Check sheet for the modelled part. Datum: model origin and axes. Units: mm. A direction names the side the tool comes from. Coordinates: 2 decimals unless noted, no trailing zeros. Write each loop counter-clockwise with the first axis right and the second up, starting at its lowest first coordinate (ties: lowest second). Pieces come first, ordered by that corner, then holes. Notation, with made-up numbers: (13.5, 18) - (61.5, 18) arc R14 ccw to (61.5, 41) - close; hole circle Ø7 at (20.5, 50.5). An arc over 180 degrees is marked (long way). Use one line per item in the form item = value. Start each with the question number.
1. Cross-section at A-A on y = 1.75. Give the number of separate pieces and of enclosed holes in the cut face, then the cut area to 3 significant figures.
2. Cross-section at B-B on y = 5.5. Record the boundary of the cut face in (x, z).
3. Scan lines: line 1 along Z through (x, y) = (-6, 1.5); line 2 along Z through (x, y) = (0, -0.6); line 3 along Y through (x, z) = (5.75, -6.5). Record each from-to range of solid material in increasing order.
4. Tool access check on faces 4 (the face through (1, 6, -13)), 5 (the face through (-0.434, -0.493, -11.348)), 6 (the face through (8.225, 1.479, -12.585)). Record the directions out of +Z, -Z, +X, -X, +Y, -Y that give a thin tool (end or side, any length) a straight path to the whole face; none if there is none.
5. Draft check along Z on faces 1 (the face through (5, 0, -11)), 2 (the face through (5.624, 1.479, -19.706)), 3 (the face through (-9.126, 1.232, -6.302)). Enter one of: +Z half, -Z half, draft (parallel to the pull), parting line (faces both ways), or undercut.
6. Go/stop test with flat-tipped pins: pin 1 Ø1.7 at (x, z) = (5.66, -18.96) entering from +Y; pin 2 Ø2 at (x, y) = (-3.5, 5) entering from +Z; pin 3 Ø0.6 at (y, z) = (6, -13.5) entering from +X. Record where each tip stops, or that it passes through.
```python
from build123d import *

# Parameters (mm, degrees)
CROQUIS1_R              = 11.5
SALIENTE_EXTRUIR1_DEPTH = 3
CROQUIS1_9_R            = 0.75
CORTAR_EXTRUIR2_DEPTH   = 3
MATRIZC2_COUNT          = 8
SALIENTE_EXTRUIR2_START = 3
CROQUIS1_11_R           = 5
SALIENTE_EXTRUIR2_DEPTH = 1.5
SALIENTE_EXTRUIR3_START = 4.5
CROQUIS1_12_R           = 2
SALIENTE_EXTRUIR3_DEPTH = 3
REDONDEO1_R             = 0.5
CROQUIS1_13_R           = 5
CROQUIS1_13_R_2         = 2
SALIENTE_EXTRUIR4_DEPTH = 1


with BuildPart() as part:
    # Croquis1 → Saliente-Extruir1 (new body)
    with BuildSketch(Plane(origin=(0, 0, 0), x_dir=(1, 0, 0), z_dir=(0, 1, 0))):
        with Locations((0, 13.3)):
            Circle(CROQUIS1_R)
    extrude(amount=SALIENTE_EXTRUIR1_DEPTH)

    # Croquis1<9> → Cortar-Extruir2 (cut)
    with BuildSketch(Plane(origin=(0, 0, 0), x_dir=(1, 0, 0), z_dir=(0, 1, 0))):
        with Locations((0, 21.3)):
            Circle(CROQUIS1_9_R)
    cortar_extruir2 = extrude(amount=CORTAR_EXTRUIR2_DEPTH, mode=Mode.SUBTRACT)

    # MatrizC2: Cortar-Extruir2 ×8 about axis
    matrizc2_axis = Axis((0, 0, -13.3), (0, 1, 0))
    for i in range(1, MATRIZC2_COUNT):
        add(cortar_extruir2.rotate(matrizc2_axis, i * 360 / MATRIZC2_COUNT), mode=Mode.SUBTRACT)

    # Croquis1<11> → Saliente-Extruir2 (add)
    with BuildSketch(Plane(origin=(0, 0, 0), x_dir=(1, 0, 0), z_dir=(0, 1, 0)).offset(SALIENTE_EXTRUIR2_START)):
        with Locations((0, 13.3)):
            Circle(CROQUIS1_11_R)
    extrude(amount=SALIENTE_EXTRUIR2_DEPTH)

    # Croquis1<12> → Saliente-Extruir3 (add)
    with BuildSketch(Plane(origin=(0, 0, 0), x_dir=(1, 0, 0), z_dir=(0, 1, 0)).offset(SALIENTE_EXTRUIR3_START)):
        with Locations((0, 13.3)):
            Circle(CROQUIS1_12_R)
        Polygon((1, 12.722649731), (1, 13.877350269), (0, 14.454700538), (-1, 13.877350269), (-1, 12.722649731), (0, 12.145299462), align=None, mode=Mode.SUBTRACT)
    extrude(amount=SALIENTE_EXTRUIR3_DEPTH)

    # Redondeo1
    redondeo1_edges = [part.edges().sort_by_distance(p)[0] for p in [
        (-11.5, 3, -13.3),
        (-5, 4.5, -13.3),
        (-2, 7.5, -13.3),
    ]]
    fillet(redondeo1_edges, radius=REDONDEO1_R)

    # Croquis1<13> → Saliente-Extruir4 (add)
    with BuildSketch(Plane(origin=(0, 0, 0), x_dir=(1, 0, 0), z_dir=(0, 1, 0))):
        with Locations((0, 13.3)):
            Circle(CROQUIS1_13_R)
        with Locations((0, 13.3)):
            Circle(CROQUIS1_13_R_2, mode=Mode.SUBTRACT)
    extrude(amount=-SALIENTE_EXTRUIR4_DEPTH)


solid = part.part
```
Final values:
q1.separate_pieces = 1
q1.enclosed_holes = 8
q1.area = 401 mm²
q2.outline = circle Ø4 at (0, -13.3); hole (-1, -13.88) - (0, -14.45) - (1, -13.88) - (1, -12.72) - (0, -12.15) - (-1, -12.72) - close
q3.line_1 = -23.11 to -19.62, -18.29 to -8.31, -6.98 to -3.49
q3.line_2 = -18.3 to -15.3, -11.3 to -8.3
q3.line_3 = 0 to 3
q4.face_4 = +Y
q4.face_5 = -Y
q4.face_6 = +Y, -Y
q5.face_1 = draft
q5.face_2 = undercut
q5.face_3 = parting line
q6.pin_1 = 3
q6.pin_2 = -9.26
q6.pin_3 = 2
